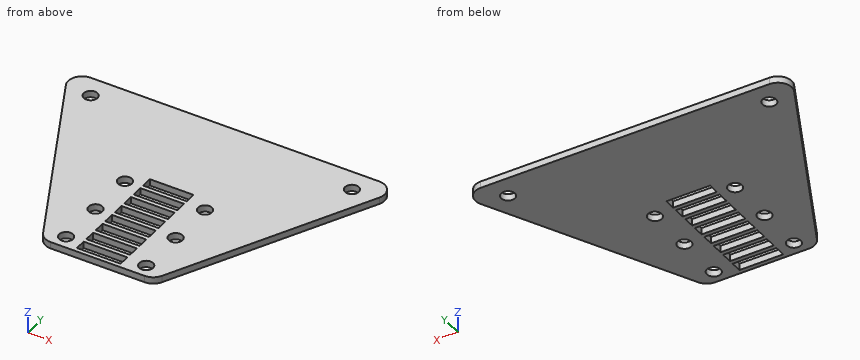
Autodesk Inventor part; units mm, degrees
ref_plane "YZ Plane" through (0, 0, 0) normal (1, 0, 0) x (0, 1, 0)
ref_plane "XZ Plane" through (0, 0, 0) normal (0, 1, 0) x (-1, 0, 0)
ref_plane "XY Plane" through (0, 0, 0) normal (0, 0, 1) x (1, 0, 0)
sketch "Sketch1" plane through (0, 0, 0) normal (0, 0, 1) x (1, 0, 0)
  line L0 (0, 0) -> (50.8, 0)
  line L1 (-50.8, 101.6) -> (101.6, 101.6)
  line L2 (50.8, 0) -> (101.6, 101.6)
  line L3 (-50.8, 101.6) -> (0, 0)
  line L4 (14.6239, 7) -> (34.6239, 7)
  line L5 (34.6239, 7) -> (34.6239, 2)
  line L6 (34.6239, 2) -> (14.6239, 2)
  line L7 (14.6239, 2) -> (14.6239, 7)
  line L8 (50.8, 0) -> (50.8, 62.4863)
  line L9 (14.6239, 14) -> (34.6239, 14)
  line L10 (34.6239, 14) -> (34.6239, 9)
  line L11 (34.6239, 9) -> (14.6239, 9)
  line L12 (14.6239, 9) -> (14.6239, 14)
  line L13 (14.6239, 21) -> (34.6239, 21)
  line L14 (34.6239, 21) -> (34.6239, 16)
  line L15 (34.6239, 16) -> (14.6239, 16)
  line L16 (14.6239, 16) -> (14.6239, 21)
  line L17 (14.6239, 28) -> (34.6239, 28)
  line L18 (34.6239, 28) -> (34.6239, 23)
  line L19 (34.6239, 23) -> (14.6239, 23)
  line L20 (14.6239, 23) -> (14.6239, 28)
  line L21 (14.6239, 35) -> (34.6239, 35)
  line L22 (34.6239, 35) -> (34.6239, 30)
  line L23 (34.6239, 30) -> (14.6239, 30)
  line L24 (14.6239, 30) -> (14.6239, 35)
  line L25 (14.6239, 42) -> (34.6239, 42)
  line L26 (34.6239, 42) -> (34.6239, 37)
  line L27 (34.6239, 37) -> (14.6239, 37)
  line L28 (14.6239, 37) -> (14.6239, 42)
  circle A0 centre (43.7057, 6.2222) radius 3.1623
  circle A1 centre (43.7057, 28) radius 3.1623
  circle A2 centre (43.7057, 49.7778) radius 3.1623
  line L29 (25.4, 0) -> (25.4, -15.6085)
  circle A3 centre (7.0943, 6.2222) radius 3.1623
  circle A4 centre (7.0943, 28) radius 3.1623
  circle A5 centre (7.0943, 49.7778) radius 3.1623
  line L30 (14.6239, 49) -> (34.6239, 49)
  line L31 (34.6239, 49) -> (34.6239, 44)
  line L32 (34.6239, 44) -> (14.6239, 44)
  line L33 (14.6239, 44) -> (14.6239, 49)
  line L34 (14.6239, 56) -> (34.6239, 56)
  line L35 (34.6239, 56) -> (34.6239, 51)
  line L36 (34.6239, 51) -> (14.6239, 51)
  line L37 (14.6239, 51) -> (14.6239, 56)
  circle A6 centre (-34.29, 91.44) radius 3.1623
  circle A7 centre (85.09, 91.44) radius 3.1623
  dimension "d0" = 50.8
  dimension "d1" = 152.4
  dimension "d2" = 101.6
  dimension "d5" = 50.8
  dimension "d6" = 20
  dimension "d7" = 5
  dimension "d8" = 2
  dimension "d11" = 7
  dimension "d16" = 6.3246
  dimension "d19" = 6.3246
  dimension "d21" = 6.3246
  dimension "d26" = 14
  dimension "d31" = 56
  dimension "d35" = 6.2222
  dimension "d36" = 6.2222
  dimension "d37" = 28
  dimension "d38" = 6.3246
  dimension "d39" = 6.3246
  dimension "d40" = 34.29
  dimension "d41" = 34.29
  dimension "d42" = 10.16
  dimension "d43" = 10.16
  dimension "d46" = 9.0818
extrude "Plate1" add sketch "Sketch1" along normal blind 3.048
fillet "Corner Round1" radius 6.35 4 edges at (101.6, 101.6, 1.524) (-50.8, 101.6, 1.524) (50.8, 0, 1.524) (0, 0, 1.524)
equation "\"d19\" = d16"
equation "\"d21\" = d19"
equation "\"d35\" = 0.111111 * d31"
equation "\"d36\" = d35"
equation "\"d37\" = 0.5 * d31"
equation "\"d41\" = d40"
equation "\"d43\" = d42"
equation "\"BendRadius\" = Thickness"
equation "\"BendReliefWidth\" = Thickness"
equation "\"BendReliefDepth\" = 0.5 * Thickness"
equation "\"CornerReliefSize\" = 4 * Thickness"
equation "\"MinimumRemnant\" = 2 * Thickness"
equation "\"TransitionRadius\" = BendRadius"
equation "\"JacobiRadiusSize\" = BendRadius"
equation "\"GapSize\" = Thickness"
equation "\"d44\" = BendRadius"
properties part number "Belt plate base"
The listing builds one solid part. Answer for the finished solid, in the listing's coordinates (mm). Coordinates: 2 decimals unless noted, no trailing zeros. Loops run counter-clockwise (first coordinate to the right, second up) from the corner with the lowest first, then second, coordinate; pieces in that order, holes last. Notation, with made-up numbers: (6.5, -40) - (54.5, -40) arc R16 cw to (54.5, -32) - close; hole circle Ø9 at (49.25, 82). An arc over 180 degrees is marked (long way). Write item = value, one per line.
1) Find the intervals of material crossed by line 1 along Y through (x, z) = (42.5, 0.3); line 2 along Y through (x, z) = (41, 2.05); line 3 along Y through (x, z) = (88, 1), in increasing order.
Responses:
line_1 = 0 to 3.3, 9.15 to 25.08, 30.92 to 46.85, 52.7 to 101.6
line_2 = 0 to 4.59, 7.86 to 26.36, 29.64 to 48.14, 51.41 to 101.6
line_3 = 74.4 to 90.2, 92.68 to 101.6
2) Section B-B (y = 90) is taken. Determine the outline of the cut face in (x, z), plus the area to 3 significant figures.
Responses:
outline = (-45, 0) - (-37.11, 0) - (-37.11, 3.05) - (-45, 3.05) - close; (-31.47, 0) - (82.27, 0) - (82.27, 3.05) - (-31.47, 3.05) - close; (87.91, 0) - (95.8, 0) - (95.8, 3.05) - (87.91, 3.05) - close
area = 395 mm^2
3) Section D-D (y = 59.5) is taken. Determine the outline of the cut face in (x, z), plus the area to 3 significant figures.
Responses:
outline = (-29.75, 0) - (80.55, 0) - (80.55, 3.05) - (-29.75, 3.05) - close
area = 336 mm^2
4) Section A-A (x = -34.29) is taken. Determine the outline of the cut face in (y, z), plus the area to 3 significant figures.
Responses:
outline = (68.58, 0) - (88.28, 0) - (88.28, 3.05) - (68.58, 3.05) - close; (94.6, 0) - (101.6, 0) - (101.6, 3.05) - (94.6, 3.05) - close
area = 81.4 mm^2
5) Section C-C (x = -13.5) is taken. Determine the outline of the cut face in (y, z).
Responses:
outline = (27, 0) - (101.6, 0) - (101.6, 3.05) - (27, 3.05) - close
6) Each of these flat-tipped pins is pushed along its axis until it touches: P1, Ø5, axis at x = -7, y = 11.5, coming from the -Z side; P2, Ø1.5, axis at y = 47, z = 2, coming from the -X side (3 decimals); P3, Ø5, axis at x = 43.71, y = 49.78, coming from the +Z side; P4, Ø0.9, axis at y = 31.5, z = 1.5, coming from the +X side (3 decimals). Where does it stop, or does it pass through?
Responses:
P1 = 0
P2 = -23.875
P3 = through
P4 = 66.775
